```python
from build123d import *

# Parameters (mm, degrees)
F0_W     = 60
F0_H     = 50
F1_DEPTH = 10
F3_DEPTH = 40
F5_DEPTH = 10.001
F7_DEPTH = 10.001


with BuildPart() as f1:
    # F0 (on Top) → F1 (new body)
    with BuildSketch(Plane.XY):
        with Locations((30, 25)):
            Rectangle(F0_W, F0_H)
    extrude(amount=F1_DEPTH)

    # F2 (on face) → F3 (join)
    with BuildSketch(Plane.XY.offset(10)):
        Polygon((0, 0), (10, 0), (10, 40), (60, 40), (60, 50), (0, 50), align=None)
    extrude(amount=F3_DEPTH)

    # F4 (on face) → F5 (cut, through all)
    with BuildSketch(Plane.YZ.offset(10)):
        Polygon((0, 10), (40, 30), (40, 50), (0, 50), align=None)
    extrude(amount=-F5_DEPTH, mode=Mode.SUBTRACT)

    # F6 (on face) → F7 (cut, through all)
    with BuildSketch(Plane.XZ.offset(-40)):
        with BuildLine():
            Line((60, 50), (50, 50))
            ThreePointArc((50, 50), (57.071068, 47.071068), (60, 40))
            Line((60, 40), (60, 50))
        make_face()
        Polygon((0, 50), (0, 30), (10, 30), (20, 30), (20, 20), (50, 20), (50, 50), align=None)
    extrude(amount=-F7_DEPTH, mode=Mode.SUBTRACT)


solid = f1.part
```
Geometry: final body of the model. Coordinates: model frame, mm. A direction names the side the tool comes from. Give positions to 0.01 mm unless a question says otherwise; leave off trailing zeros. Loops run counter-clockwise (first coordinate to the right, second up) from the corner with the lowest first, then second, coordinate; pieces in that order, holes last. Notation, with made-up numbers: (12.5, -8.75) -> (21.5, -8.75) arc R23 ccw to (21.5, 27.25) -> close; hole circle Ø10 at (-29.75, 62). An arc over 180 degrees is marked (long way). Return JSON: item names as keys, results as strings.
Item 1: Mould query, pull axis X, two halves, no side actions, for faces 4 (the cylindrical face through (56.99, 44.93, 47.15)), 5 (the flat face through (35, 45, 20)), 6 (the flat face through (10, 45, 30)), 7 (the flat face through (50, 45, 35)). Classes: released by +X, released by -X, zero draft, split by the parting line, or undercut.
Filled in:
{"face 4": "released by +X", "face 5": "undercut", "face 6": "zero draft", "face 7": "undercut"}
Item 2: Section A-A, the plane z = 22. Output: boundary loops of the cut face in (x, y).
Filled in:
{"outline": "(0, 24) -> (10, 24) -> (10, 40) -> (20, 40) -> (20, 50) -> (0, 50) -> close; (50, 40) -> (60, 40) -> (60, 50) -> (50, 50) -> close"}
Item 3: Section B-B, the plane x = 7. Output: boundary loops of the cut face in (y, z).
Filled in:
{"outline": "(0, 0) -> (50, 0) -> (50, 30) -> (40, 30) -> (0, 10) -> close"}
Item 4: Pin query (flat end, axial travel): P1, Ø8, axis at x = 30.5, y = 45.5, coming from the +Z side; P2, Ø12, axis at x = 23, y = 17, coming from the +Z side; P3, Ø5, axis at x = 13.5, y = 45, coming from the +Z side. Return the tip coordinate at first contact, or that it passes through.
Filled in:
{"P1": "z = 20", "P2": "z = 10", "P3": "z = 30"}
Item 5: Access query for faces 1 (the flat face through (20, 45, 25)), 2 (the flat face through (0, 31, 11)), 3 (the flat face through (10, 29, 15)). Directions: +Z, -Z, +X, -X, +Y, -Y. A direction counts if a zero-diameter tool reaches every point of the face in a straight line with its end or side. Return the directions, or none.
Filled in:
{"face 1": "+Z, +Y, -Y", "face 2": "+Z, -Z, -X, +Y, -Y", "face 3": "+Z, +X, -Y"}
Item 6: Section D-D, the plane z = 12.5. Output: boundary loops of the cut face in (x, y).
Filled in:
{"outline": "(0, 5) -> (10, 5) -> (10, 40) -> (60, 40) -> (60, 50) -> (0, 50) -> close"}
Item 7: Line query: line 1 (Z direction, x = 32, y = 42.5); line 2 (Y direction, x = 11, z = 28); line 3 (X direction, y = 38, z = 15). Output: solid intervals per line, ascending.
Filled in:
{"line 1": "0 to 20", "line 2": "40 to 50", "line 3": "0 to 10"}
Item 8: Section C-C, the plane y = 44.5. Output: boundary loops of the cut face in (x, z), plus the area to 3 significant figures.
Filled in:
{"outline": "(0, 0) -> (60, 0) -> (60, 40) arc R10 ccw to (50, 50) -> (50, 20) -> (20, 20) -> (20, 30) -> (0, 30) -> close", "area": "1,680 mm^2"}
